The listing builds one solid part. Answer for the finished solid, in the listing's coordinates (mm). Round coordinates to 2 decimals unless told otherwise and drop trailing zeros. Write each loop counter-clockwise with the first axis right and the second up, starting at its lowest first coordinate (ties: lowest second). Pieces come first, ordered by that corner, then holes. Notation, with made-up numbers: M -3,-8 L 38,-8 A15 ccw 38,6 Z; hole C -7,-4 d5. An arc over 180 degrees is marked long. Put each result on its own line as item: value. Start each with the question number.
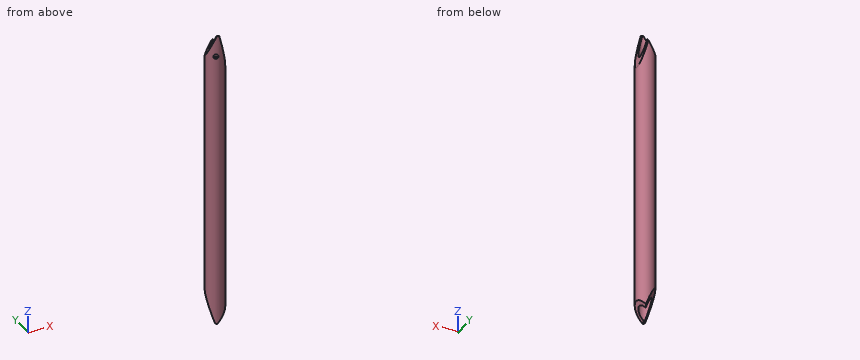
Autodesk Inventor part; units mm, degrees
ref_plane "Start Plane" through (0, 0, -4.8828) normal (0, 0, 1) x (1, 0, 0)
ref_plane "End Plane" through (0, 0, 346.6281) normal (0, 0, 1) x (1, 0, 0)
ref_plane "Work Plane4" through (8.6921, -6.185, 361.8082) normal (-0.7364, 0.524, 0.4281) x (0.6203, 0.2702, 0.7364)
ref_plane "Start Plane" through (0, 0, -4.8828) normal (0, 0, 1) x (1, 0, 0)
ref_plane "End Plane" through (0, 0, 346.6281) normal (0, 0, 1) x (1, 0, 0)
sketch "Sketch" plane through (0, 0, 0) normal (0, 0, 1) x (1, 0, 0)
  circle A0 centre (0, 0) radius 6.9342
  circle A1 centre (0, 0) radius 10.668
  dimension "d0" = 21.336
  dimension "d1" = 3.7338
extrude "Body" add sketch "Sketch" along normal up to surface (351.5109 mm away) from surface at -4.8828
sketch "Sketch3" plane through (0, 0, 0) normal (0, 0, 1) x (1, 0, 0)
  line L0 (0, 0) -> (10, 0)
ref_plane "Work Plane3" through (0, 0, 0) normal (0, -1, 0) x (1, 0, 0)
sketch "Sketch4" plane through (0, 0, 0) normal (0, -1, 0) x (1, 0, 0)
  line L0 (-2, -4.8828) -> (12, -4.8828)
  line L1 (-2, 346.6281) -> (12, 346.6281)
  dimension "d7" = 351.5109
ref_plane "Work Plane4" through (8.6921, -6.185, 361.8082) normal (-0.7364, 0.524, 0.4281) x (0.6203, 0.2702, 0.7364)
split "Split1" plane through (8.6921, -6.185, 361.8082) removes the side toward (-0.7364, 0.524, 0.4281)
ref_plane "Work Plane5" through (-3.8378, -9.9538, 346.6526) normal (0.2044, 0.5302, 0.8228) x (0.9771, -0.0595, -0.2044)
split "Split2" plane through (-3.8378, -9.9538, 346.6526) removes the side toward (0.2044, 0.5302, 0.8228)
ref_plane "Work Plane6" through (-10.6086, -1.1246, 380.9088) normal (0.9633, 0.1021, 0.2483) x (0.2566, -0.0788, -0.9633)
split "Split3" plane through (-10.6086, -1.1246, 380.9088) removes the side toward (0.9633, 0.1021, 0.2483)
ref_plane "Work Plane7" through (8.6921, -6.185, -30.4674) normal (-0.769, 0.5472, -0.3305) x (0.1167, 0.6285, 0.769)
split "Split4" plane through (8.6921, -6.185, -30.4674) removes the side toward (-0.769, 0.5472, -0.3305)
ref_plane "Work Plane8" through (-10.6086, -1.1246, -13.2489) normal (0.7745, 0.0821, -0.6272) x (-0.6091, -0.1706, -0.7745)
split "Split5" plane through (-10.6086, -1.1246, -13.2489) removes the side toward (0.7745, 0.0821, -0.6272)
ref_plane "Work Plane9" through (2.6801, -10.3259, -5.6452) normal (-0.1175, 0.4527, -0.8839) x (0.8811, 0.4581, 0.1175)
split "Split6" plane through (2.6801, -10.3259, -5.6452) removes the side toward (-0.1175, 0.4527, -0.8839)
ref_plane "Work Plane10" through (-46.7913, -3.422, 233.5882) normal (-0.5112, -0.8523, 0.111) x (0.8583, -0.5129, 0.0149)
sketch "Sketch5" plane through (-46.7913, -3.422, 233.5882) normal (-0.5112, -0.8523, 0.111) x (0.8583, -0.5129, 0.0149)
  circle A0 centre (41.1209, 88.8492) radius 4
  point P0 (34.9285, -229.6953)
hole "Hole1" at (-7.5645, -15.3691, 322.4906) direction (0.5112, 0.8523, -0.111) diameter 5.4 depth 20 tip angle 118
equation "\"d0\" = G_H"
equation "\"d1\" = G_T"
equation "\"d2\" = G_L"
equation "\"G_H\" = 21.336"
equation "\"G_T\" = 3.7338"
equation "\"G_L\" = 351.51086"
equation "\"G_OFFSET_START\" = 4.88279"
equation "\"G_OFFSET_END\" = 7.34335"
equation "\"d4\" = -G_OFFSET_START"
equation "\"d5\" = G_OFFSET_END + B_L"
equation "\"B_L\" = 339.28473"
properties part number "ANSI - 1/2 x 0.147 - 13.839" material "Steel, Mild"
Item 1: Section A-A (y = 0) is taken. Give the vertices of the cut face in (x, z), and give its area (3 significant figures).
Item 2: Section B-B (z = 250.5) is taken. Give the vertices of the cut face in (x, y).
Item 3: Section C-C (z = 27.5) is taken. Give the vertices of the cut face in (x, y).
Item 4: Flat-ended cylindrical pins translate along their axes: pin 1 (5 mm diameter, centred on x = 4.5, z = 149, fed in from -Y); pin 2 (3 mm diameter, centred on x = 6, z = 174.5, fed in from +Y); pin 3 (8 mm diameter, centred on x = 7, y = 0.5, fed in from -Z). Find the tip coordinate at first contact, or state that the pin passes through.
Item 5: Consider line 1 along X through (y, z) = (0, 122); line 2 along Y through (x, z) = (0.75, 70.5). Determine where each line is inside the solid, lowest interval first. Write a range as [from, to].
Output values:
1. outline: M -10.67,24.82 L -6.93,16.13 L -6.93,327.36 L -10.67,320.94 Z; M 6.93,8.56 L 10.67,13.17 L 10.67,297.9 L 6.93,312.39 Z
1. area: 2,230 mm^2
2. outline: C 0,0 d21.34; hole C 0,0 d13.87
3. outline: M -10.51,1.84 A10.67 ccw long -5.19,9.32 Z; hole C 0,0 d13.87
4. pin 1: stops at y = -10.48
4. pin 2: stops at y = 9.67
4. pin 3: stops at z = 7.03
5. line 1: x = [-10.67, -6.93], [6.93, 10.67]
5. line 2: y = [-10.64, -6.89], [6.89, 10.64]
